Input: part model. Units: mm. Frame: model coordinates. Coordinates: 2 decimals unless noted, no trailing zeros. Loops run counter-clockwise (first coordinate to the right, second up) from the corner with the lowest first, then second, coordinate; pieces in that order, holes last.
Item 1: Section D-D on x = -42.5. Return loops of the section in (y, z).
Item 2: Contact query for flat-ended pins moving along their axis: P1, Ø0.5, axis at y = 0.5, z = 4.5, coming from the -X side; P2, Ø0.5, axis at x = -17.5, y = 0.5, coming from the -Z side. Output: stop coordinate, or through.
Item 3: Section A-A on z = 19.25. Return loops of the section in (x, y), and give its area (3 significant figures).
Item 4: Section C-C on y = 0.35. Give the number of separate pieces and of enclosed holes in the cut face, and give its area (3 significant figures).
Item 5: Section B-B on z = 12.75. Return loops of the section in (x, y), and give its area (3 significant figures).
Item 6: Ray query, line 1 along X through (y, z) = (0.1, 11.75); line 2 along X through (y, z) = (0.95, 10.5); line 3 along X through (y, z) = (0.6, 19.5). Return the intervals inside material, ascending.
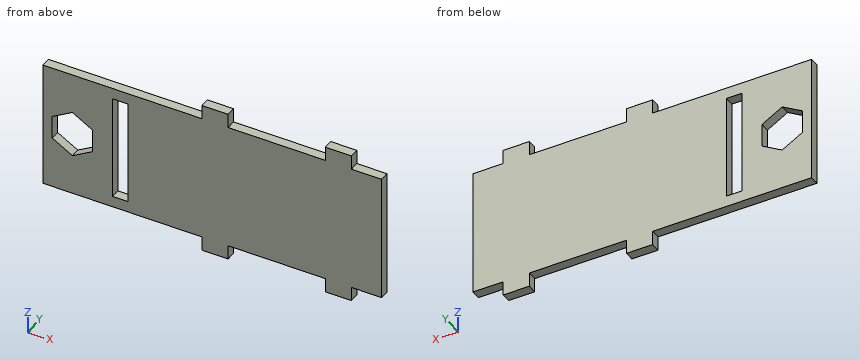
```python
from build123d import *

# Parameters (mm, degrees)
SKETCH1_W              = 35.7
SKETCH1_H              = 13.45
BOSS_EXTRUDE1_DEPTH    = 1
SKETCH2_W              = 2.75
SKETCH2_H              = 1.5
BOSS_EXTRUDE2_DEPTH    = 1
SKETCH3_W              = 1.65
SKETCH3_H              = 11.1
ADAPTER_PCB_HOLE_DEPTH = 1
CUT_EXTRUDE2_DEPTH     = 1


with BuildPart() as part:
    # Sketch1 → Boss-Extrude1 (new body)
    with BuildSketch(Plane(origin=(0, 0, 0), x_dir=(1, 0, 0), z_dir=(0, 1, 0))):
        with Locations((-32.948423651, -12.055454233)):
            Rectangle(SKETCH1_W, SKETCH1_H)
    extrude(amount=BOSS_EXTRUDE1_DEPTH)

    # Sketch2 → Boss-Extrude2 (add)
    with BuildSketch(Plane(origin=(0, 0, 0), x_dir=(1, 0, 0), z_dir=(0, 1, 0))):
        with Locations((-32.658423651, -4.580454233)):
            Rectangle(SKETCH2_W, SKETCH2_H)
        with Locations((-32.658423651, -19.530454233)):
            Rectangle(SKETCH2_W, SKETCH2_H)
        with Locations((-19.658423651, -4.580454233)):
            Rectangle(SKETCH2_W, SKETCH2_H)
        with Locations((-19.658423651, -19.530454233)):
            Rectangle(SKETCH2_W, SKETCH2_H)
    extrude(amount=BOSS_EXTRUDE2_DEPTH)

    # Sketch3 → adapter_PCB_hole (cut)
    with BuildSketch(Plane(origin=(0, 0, 0), x_dir=(-1, 0, 0), z_dir=(0, -1, 0))):
        with Locations((42.643423651, -12.055454233)):
            Rectangle(SKETCH3_W, SKETCH3_H)
    extrude(amount=-ADAPTER_PCB_HOLE_DEPTH, mode=Mode.SUBTRACT)

    # Sketch4 → Cut-Extrude2 (cut)
    with BuildSketch(Plane(origin=(0, 0, 0), x_dir=(-1, 0, 0), z_dir=(0, -1, 0))):
        Polygon((49.823423651, -13.282323555), (49.823423651, -10.828584911), (47.698423651, -9.601715589), (45.573423651, -10.828584911), (45.573423651, -13.282323555), (47.698423651, -14.509192877), align=None)
    extrude(amount=-CUT_EXTRUDE2_DEPTH, mode=Mode.SUBTRACT)


solid = part.part
```
Results found:
1. outline: (0, 5.33) - (1, 5.33) - (1, 6.51) - (0, 6.51) - close; (0, 17.61) - (1, 17.61) - (1, 18.78) - (0, 18.78) - close
2. P1: stops at x = -34.03
2. P2: stops at z = 5.33
3. outline: (-34.03, 0) - (-31.28, 0) - (-31.28, 1) - (-34.03, 1) - close; (-21.03, 0) - (-18.28, 0) - (-18.28, 1) - (-21.03, 1) - close
3. area: 5.50 mm2
4. separate pieces: 1
4. enclosed holes: 2
4. area: 463 mm2
5. outline: (-50.8, 0) - (-49.82, 0) - (-49.82, 1) - (-50.8, 1) - close; (-45.57, 0) - (-43.47, 0) - (-43.47, 1) - (-45.57, 1) - close; (-41.82, 0) - (-15.1, 0) - (-15.1, 1) - (-41.82, 1) - close
5. area: 29.8 mm2
6. line 1: x = -50.8 to -49.82, -45.57 to -43.47, -41.82 to -15.1
6. line 2: x = -50.8 to -49.25, -46.14 to -43.47, -41.82 to -15.1
6. line 3: x = -34.03 to -31.28, -21.03 to -18.28
